Autodesk Inventor part; units mm, degrees
ref_plane "YZ Plane" through (0, 0, 0) normal (1, 0, 0) x (0, 1, 0)
ref_plane "XZ Plane" through (0, 0, 0) normal (0, 1, 0) x (-1, 0, 0)
ref_plane "XY Plane" through (0, 0, 0) normal (0, 0, 1) x (1, 0, 0)
sketch "Sketch1" plane through (0, 0, 0) normal (0, 0, 1) x (1, 0, 0)
  circle A0 centre (0, 0) radius 80 construction
  line L0 (0, 80) -> (20, 80)
  line L1 (0, -80) -> (20, -80)
  line L2 (20, -80) -> (20, 80)
  arc A1 (0, 80) -> (0, -80) centre (0, 0) ccw
  circle A2 centre (0, 0) radius 7
  dimension "d0" = 160
  dimension "d1" = 20
  dimension "d3" = 14
extrude "Extrusion1" add sketch "Sketch1" along normal blind 120
sketch "Sketch2" plane through (20, -80, 0) normal (1, 0, 0) x (0, 0, -1)
  line L0 (-120, 160) -> (-120, 0)
  line L1 (-120, 55.875) -> (0, 55.875) construction
  line L2 (0, 0) -> (0, 160)
  line L3 (-120, 0) -> (-120, 160)
  circle A0 centre (-42.5, 55.875) radius 2.5
  circle A1 centre (-77.5, 55.875) radius 2.5
  point P0 (0, 80)
  dimension "d6" = 24.125
  dimension "d7" = 5
  dimension "d8" = 5
  dimension "d9" = 42.5
  dimension "d10" = 35
extrude "Extrusion2" cut sketch "Sketch2" against normal blind 35
sketch "Sketch3" plane through (0, 0, 120) normal (0, 0, 1) x (1, 0, 0)
  circle A0 centre (0, 35) radius 2.5
  circle A1 centre (-30.3109, 17.5) radius 2.5
  circle A2 centre (-30.3109, -17.5) radius 2.5
  circle A3 centre (0, -35) radius 2.5
  circle A4 centre (30.3109, -17.5) radius 2.5
  circle A5 centre (30.3109, 17.5) radius 2.5
  point P0 (0, 0)
  dimension "d14" = 5
  dimension "d15" = 35
  dimension "d18" = 360
extrude "Extrusion3" cut sketch "Sketch3" against normal through all
properties part number "AA004" material "ABS Plastic"
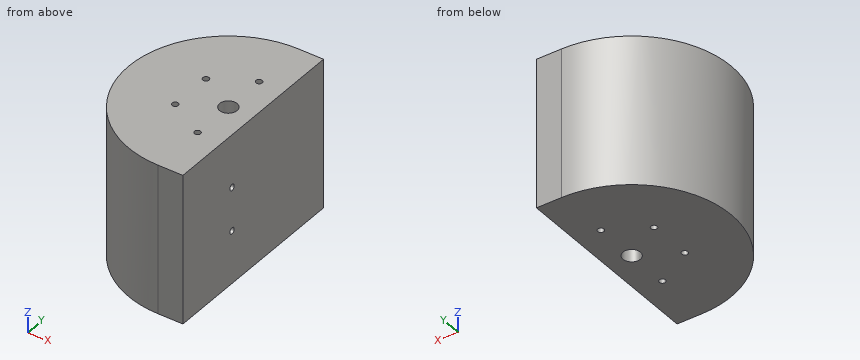
Check sheet for the modelled part. Datum: model origin and axes. Units: mm. Round coordinates to 2 decimals unless told otherwise and drop trailing zeros. Loops run counter-clockwise (first coordinate to the right, second up) from the corner with the lowest first, then second, coordinate; pieces in that order, holes last. Notation, with made-up numbers: (-29.5, -26) - (26.5, -26) arc R20 cw to (26.5, 3) - close; hole circle Ø8 at (-3.5, 89). An arc over 180 degrees is marked (long way). Answer as CSV lines item,"result". Start each with the question number.
Item 1: Section check A-A (y = 0). Record the boundary of the cut face in (x, z), and give its area (3 significant figures).
Item 2: Section check D-D (y = -17.5). Record the boundary of the cut face in (x, z).
Item 3: Scan lines: line 1 (Y direction, x = 0, z = 29.5); line 2 (Y direction, x = 2, z = 42); line 3 (X direction, y = -19, z = 33.5). Record each from-to range of solid material in increasing order. Write a range as [from, to].
Item 4: Section check C-C (z = 42.5). Record the boundary of the cut face in (x, y) (3 decimals).
Item 5: Depth check by flat-ended pin: P1, Ø5, axis at x = -53.5, z = 97, coming from the +Y side; P2, Ø6, axis at x = -32.5, z = 46.5, coming from the -Y side; P3, Ø5, axis at x = -25, z = 86, coming from the +Y side. Enter the tip coordinate at first touch or a pass-through.
Item 6: Section check B-B (z = 54.5). Record the boundary of the cut face in (x, y), and give its area (3 significant figures).
Report:
1,outline,"(-80, 0) - (-7, 0) - (-7, 120) - (-80, 120) - close; (7, 0) - (20, 0) - (20, 120) - (7, 120) - close"
1,area,"10,300 mm2"
2,outline,"(-78.06, 0) - (-32.81, 0) - (-32.81, 120) - (-78.06, 120) - close; (-27.81, 0) - (20, 0) - (20, 120) - (-27.81, 120) - close"
3,line 1,"y = [-80, -37.5], [-32.5, -7], [7, 32.5], [37.5, 80]"
3,line 2,"y = [-80, -36.5], [-33.5, -26.57], [-21.68, -6.71], [6.71, 33.5], [36.5, 80]"
3,line 3,"x = [-77.71, -32.31], [-28.31, 20]"
4,outline,"(-15, -26.625) - (-15, -21.625) - (20, -21.625) - (20, 80) - (0, 80) arc R80 ccw to (0, -80) - (20, -80) - (20, -26.625) - close; hole circle Ø5 at (-30.311, -17.5); hole circle Ø5 at (-30.311, 17.5); hole circle Ø14 at (0, 0); hole circle Ø5 at (0, -35); hole circle Ø5 at (0, 35)"
5,P1,"stops at y = 61.64"
5,P2,"stops at y = -74.36"
5,P3,"stops at y = 76.77"
6,outline,"(0, -80) - (20, -80) - (20, 80) - (0, 80) arc R80 ccw to start; hole circle Ø5 at (-30.31, -17.5); hole circle Ø5 at (-30.31, 17.5); hole circle Ø14 at (0, 0); hole circle Ø5 at (0, -35); hole circle Ø5 at (0, 35)"
6,area,"13,000 mm2"
